Build history of the part. All positions in model axes, mm. A direction names the side the tool comes from. Round coordinates to 2 decimals unless told otherwise and drop trailing zeros. Order: outer loops, then holes, each group sorted by start corner. A loop starts at its lowest first (then second) coordinate and runs counter-clockwise, first axis right, second up. Notation, with made-up numbers: (79.25, -5.75) -> (98.25, -5.75) arc R24 cw to (98.25, 30.25) -> close; hole circle Ø9 at (-21, 74.25). An arc over 180 degrees is marked (long way). Answer as a JSON object with one key per item and string values.
from build123d import *

# Parameters (mm, degrees)
BOSS_EXTRUDE1_DEPTH = 4.5
SKETCH2_R           = 7.5
CUT_EXTRUDE1_DEPTH  = 50.942466899
SKETCH3_R           = 4
BOSS_EXTRUDE2_DEPTH = 7
BOSS_EXTRUDE3_DEPTH = 4.5
FILLET1_R           = 10
CUT_EXTRUDE4_DEPTH  = 62.754464971
SKETCH9_R           = 1
CUT_EXTRUDE5_DEPTH  = 62.182594482
SKETCH10_R          = 1.7
CUT_EXTRUDE6_DEPTH  = 2.4
CUT_EXTRUDE7_DEPTH  = 4.5
FILLET2_R           = 10
CUT_EXTRUDE8_DEPTH  = 51.658168147
SKETCH20_R          = 1
BOSS_EXTRUDE4_DEPTH = 4.5
SKETCH21_R          = 2
CUT_EXTRUDE9_DEPTH  = 3


with BuildPart() as part:
    # Sketch1 → Boss-Extrude1 (new body)
    with BuildSketch(Plane.XY):
        with BuildLine():
            Line((10.483870968, 22.695560128), (36.032258065, 10.893868862))
            ThreePointArc((36.032258065, 10.893868862), (43, 0), (36.032258065, -10.893868862))
            Line((36.032258065, -10.893868862), (10.483870968, -22.695560128))
            ThreePointArc((10.483870968, -22.695560128), (-25, 0), (10.483870968, 22.695560128))
        make_face()
    extrude(amount=BOSS_EXTRUDE1_DEPTH)

    # Sketch2 → Cut-Extrude1 (cut, through all)
    with BuildSketch(Plane.XY.offset(4.5)):
        with Locations((31, 0)):
            Circle(SKETCH2_R)
    extrude(amount=-CUT_EXTRUDE1_DEPTH, mode=Mode.SUBTRACT)

    # Sketch3 → Boss-Extrude2 (add)
    with BuildSketch(Plane.XY.offset(4.5)):
        Circle(SKETCH3_R)
    extrude(amount=BOSS_EXTRUDE2_DEPTH)

    # Sketch4 → Boss-Extrude3 (add)
    with BuildSketch(Plane(origin=(0, 0, 0), x_dir=(-1, 0, 0), z_dir=(0, 0, -1))):
        with BuildLine():
            Line((-36.032258065, 10.893868862), (-56.032258065, 10.893868862))
            Line((-56.032258065, 10.893868862), (-56.032258065, -10.893868862))
            Line((-56.032258065, -10.893868862), (-36.032258065, -10.893868862))
            ThreePointArc((-36.032258065, -10.893868862), (-43, 0), (-36.032258065, 10.893868862))
        make_face()
        with BuildLine():
            Line((22.501635968, 10.893868862), (42.501635968, 10.893868862))
            Line((42.501635968, 10.893868862), (42.501635968, -10.893868862))
            Line((42.501635968, -10.893868862), (22.501635968, -10.893868862))
            ThreePointArc((22.501635968, -10.893868862), (25, 0), (22.501635968, 10.893868862))
        make_face()
    extrude(amount=-BOSS_EXTRUDE3_DEPTH)

    # Fillet1
    fillet1_edges = [part.edges().sort_by_distance(p)[0] for p in [
        (56.032258065, 10.893868862, 2.25),
        (56.032258065, -10.893868862, 2.25),
        (-42.501635968, -10.893868862, 2.25),
        (-42.501635968, 10.893868862, 2.25),
    ]]
    fillet(fillet1_edges, radius=FILLET1_R)

    # Sketch8 → Cut-Extrude4 (cut, through all)
    with BuildSketch(Plane.XY.offset(4.5)):
        with BuildLine():
            Line((56.032258065, 0.893868862), (56.032258065, -0.893868862))
            ThreePointArc((56.032258065, -0.893868862), (55.873267798, -2.669967796), (55.401352579, -4.389590243))
            Line((55.401352579, -4.389590243), (55.401352579, 4.389590243))
            ThreePointArc((55.401352579, 4.389590243), (55.873267798, 2.669967796), (56.032258065, 0.893868862))
        make_face()
        with BuildLine():
            Line((-42.501635968, -0.893868862), (-42.501635968, 0.893868862))
            ThreePointArc((-42.501635968, 0.893868862), (-42.342645701, 2.669967796), (-41.870730482, 4.389590243))
            Line((-41.870730482, 4.389590243), (-41.870730482, -4.389590243))
            ThreePointArc((-41.870730482, -4.389590243), (-42.342645701, -2.669967796), (-42.501635968, -0.893868862))
        make_face()
    extrude(amount=-CUT_EXTRUDE4_DEPTH, mode=Mode.SUBTRACT)

    # Sketch9 → Cut-Extrude5 (cut, through all)
    with BuildSketch(Plane.XY.offset(4.5)):
        with Locations((-8.154330676, 12.589951995)):
            Circle(SKETCH9_R)
        with Locations((12.589951995, 8.154330676)):
            Circle(SKETCH9_R)
        with Locations((8.154330676, -12.589951995)):
            Circle(SKETCH9_R)
        with Locations((-12.589951995, -8.154330676)):
            Circle(SKETCH9_R)
    extrude(amount=-CUT_EXTRUDE5_DEPTH, mode=Mode.SUBTRACT)

    # Sketch10 → Cut-Extrude6 (cut)
    with BuildSketch(Plane.XY.offset(4.5)):
        with Locations((-8.154330676, 12.589951995)):
            Circle(SKETCH10_R)
        with Locations((12.589951995, 8.154330676)):
            Circle(SKETCH10_R)
        with Locations((8.154330676, -12.589951995)):
            Circle(SKETCH10_R)
        with Locations((-12.589951995, -8.154330676)):
            Circle(SKETCH10_R)
    extrude(amount=-CUT_EXTRUDE6_DEPTH, mode=Mode.SUBTRACT)

    # Sketch11 → Cut-Extrude7 (cut)
    with BuildSketch(Plane(origin=(0, 0, 0), x_dir=(-1, 0, 0), z_dir=(0, 0, -1))):
        with BuildLine():
            Line((-40.960235838, 14.646128502), (-73.67178465, 18.9155259))
            Line((-73.67178465, 18.9155259), (-68.640309048, -15.675868866))
            Line((-68.640309048, -15.675868866), (-41.444996676, -13.212200821))
            ThreePointArc((-41.444996676, -13.212200821), (-43.493415761, 0.756825882), (-40.960235838, 14.646128502))
        make_face()
    extrude(amount=-CUT_EXTRUDE7_DEPTH, mode=Mode.SUBTRACT)

    # Fillet2
    # the kernel refuses this fillet: 10 mm, written as the material it takes off along each edge
    with BuildSketch(Plane(origin=(42.113817462, -10.893868862, 28.001897109), x_dir=(0.1443560651040101, 0.9895258088941827, 0), z_dir=(0, 0, -1))) as fillet2_piece_1:
        with BuildLine():
            CenterArc((8.32021185, -9.941449502), FILLET2_R, 83.796810377, 73.10182949)
            Line((-0.877909984, -6.017859982), (-1.061872421, -5.939388192))
            ThreePointArc((-1.061872421, -5.939388192), (-0.636860154, -2.980058778), (-0.197905162, 0.028871213))
            Line((-0.197905162, 0.028871213), (-0.02161094, 0.19882899))
            ThreePointArc((-0.02161094, 0.19882899), (4.700379422, 0.454694668), (9.422369784, 0.19882899))
            Line((9.422369784, 0.19882899), (9.400758844, 0))
        make_face()
    extrude(amount=51.503794219, mode=Mode.SUBTRACT)
    with BuildSketch(Plane(origin=(42.113817462, 10.893868862, 28.001897109), x_dir=(-1, 0, 0), z_dir=(0, 0, -1))) as fillet2_piece_2:
        with BuildLine():
            CenterArc((8.636247816, -9.668172893), FILLET2_R, 104.801368002, 73.10182949)
            Line((-1.357056556, -9.302293499), (-1.556922643, -9.294975911))
            ThreePointArc((-1.556922643, -9.294975911), (-1.128460387, -4.585508816), (-0.193626747, 0.050086753))
            Line((-0.193626747, 0.050086753), (0, 0.2))
            ThreePointArc((0, 0.2), (3.040779699, 0.2), (6.030465629, 0.193363458))
            Line((6.030465629, 0.193363458), (6.081559398, 0))
        make_face()
    extrude(amount=51.503794219, mode=Mode.SUBTRACT)

    # Sketch12 → Cut-Extrude8 (cut, through all)
    with BuildSketch(Plane.XY.offset(4.5)):
        with BuildLine():
            Line((-22.501635968, 10.893868862), (-42.592674389, 14.819498464))
            Line((-42.592674389, 14.819498464), (-48.148078041, -13.612584929))
            Line((-48.148078041, -13.612584929), (-27.427309778, -14.315310761))
            Line((-27.427309778, -14.315310761), (-22.501635968, -10.893868862))
            ThreePointArc((-22.501635968, -10.893868862), (-25, 0), (-22.501635968, 10.893868862))
        make_face()
    extrude(amount=-CUT_EXTRUDE8_DEPTH, mode=Mode.SUBTRACT)

    # Sketch20 → Boss-Extrude4 (add)
    with BuildSketch(Plane.XY.offset(4.5)):
        with BuildLine():
            Line((55.798644786, -13.311457412), (55.798644786, 13.726073795))
            Line((55.798644786, 13.726073795), (30.798644786, 13.726073795))
            Line((30.798644786, 13.726073795), (30.798644786, 13.311457412))
            Line((30.798644786, 13.311457412), (36.032258065, 10.893868862))
            ThreePointArc((36.032258065, 10.893868862), (41.287575846, 7.470998455), (43.470874018, 1.591575362))
            ThreePointArc((43.470874018, 1.591575362), (43.5, 0), (43.470874018, -1.591575362))
            ThreePointArc((43.470874018, -1.591575362), (41.287575846, -7.470998455), (36.032258065, -10.893868862))
            Line((36.032258065, -10.893868862), (30.798644786, -13.311457412))
            Line((30.798644786, -13.311457412), (55.798644786, -13.311457412))
        make_face()
        with Locations((47.197816856, -7.773648876)):
            Circle(SKETCH20_R, mode=Mode.SUBTRACT)
        with Locations((47.197816856, 8.226351124)):
            Circle(SKETCH20_R, mode=Mode.SUBTRACT)
    extrude(amount=-BOSS_EXTRUDE4_DEPTH)

    # Sketch21 → Cut-Extrude9 (cut)
    with BuildSketch(Plane.XY.offset(4.5)):
        with Locations((47.197816856, 8.226351124)):
            Circle(SKETCH21_R)
        with Locations((47.197816856, -7.773648876)):
            Circle(SKETCH21_R)
    extrude(amount=-CUT_EXTRUDE9_DEPTH, mode=Mode.SUBTRACT)


solid = part.part
1) Cut at B-B, the plane x = 27.5. Give the cut face in (y, z).
Checked values:
{"outline": "(-14.84, 0) -> (-6.63, 0) -> (-6.63, 4.5) -> (-14.84, 4.5) -> close; (6.63, 0) -> (14.84, 0) -> (14.84, 4.5) -> (6.63, 4.5) -> close"}
2) Probe L1, parallel to X at y = 13.5, z = 1; L2, parallel to X at y = 9, z = 1.25; L3, parallel to Y at x = 31, z = 1.1. List the from-to ranges inside material, lowest first. Write a range as from..to.
Checked values:
{"L1": "x = -21.04..-8.57, -7.74..30.39, 30.8..55.8", "L2": "x = -23.32..12.06, 13.12..46.56, 47.83..55.8", "L3": "y = -13.31..-7.5, 7.5..13.73"}
3) Pull direction X, two halves, no side cores. Call faces 1 (the face through (-0.867, -3.905, 7.951)), 2 (the face through (10.89, 8.23, 3.32)), 3 (the face through (15, 0, 4.5)): pulls with the +X half, pulls with the -X half, needs draft (parallel to the pull), parting line crosses it, or undercut.
Checked values:
{"face 1": "parting line crosses it", "face 2": "undercut", "face 3": "needs draft"}
4) Cut at A-A, the plane y = 0. Give the cut face in (x, z), plus the area to 3 significant figures.
Checked values:
{"outline": "(-25, 0) -> (23.5, 0) -> (23.5, 4.5) -> (4, 4.5) -> (4, 11.5) -> (-4, 11.5) -> (-4, 4.5) -> (-25, 4.5) -> close; (38.5, 0) -> (55.8, 0) -> (55.8, 4.5) -> (38.5, 4.5) -> close", "area": "352 mm²"}
5) Cut at C-C, the plane z = 3. Give the cut face in (x, y), plus the area to 3 significant figures.
Checked values:
{"outline": "(10.48, -22.7) -> (30.8, -13.31) -> (55.8, -13.31) -> (55.8, 13.73) -> (30.8, 13.73) -> (30.8, 13.31) -> (10.48, 22.7) arc R25 ccw (long way) to start; hole circle Ø3.4 at (-12.59, -8.15); hole circle Ø3.4 at (-8.15, 12.59); hole circle Ø3.4 at (8.15, -12.59); hole circle Ø3.4 at (12.59, 8.15); hole circle Ø15 at (31, 0); hole circle Ø4 at (47.2, -7.77); hole circle Ø4 at (47.2, 8.23)", "area": "2,660 mm²"}
6) Cut at D-D, the plane x = 0. Give the cut face in (y, z).
Checked values:
{"outline": "(-25, 0) -> (25, 0) -> (25, 4.5) -> (4, 4.5) -> (4, 11.5) -> (-4, 11.5) -> (-4, 4.5) -> (-25, 4.5) -> close"}
7) Which spindle directions (+Z, -Z, +X, -X, +Y, -Y) get a long thin tool onto all of the face, cutting with end or side? Do faces 4 (the face through (-8.285, 13.581, 1.065)), 5 (the face through (43, -13.311, 2)), 6 (the face through (46.764, -9.726, 3.021)), 7 (the face through (43, 13.726, 2)). Say none if no direction does.
Checked values:
{"face 4": "+Z, -Z", "face 5": "+Z, -Z, +X, -Y", "face 6": "+Z", "face 7": "+Z, -Z, +X, +Y"}
8) Flat gauge pins, fed straight in: pin 1 Ø2.5 at (x, y) = (47.2, -7.77) entering from +Z; pin 2 Ø6 at (x, y) = (5, 18.5) entering from +Z; pin 3 Ø1.6 at (x, y) = (12.59, 8.15) entering from -Z; pin 4 Ø12 at (x, y) = (24.5, -19) entering from -Z. Where does each tip first touch, or does it go through?
Checked values:
{"pin 1": "stops at z = 1.5", "pin 2": "stops at z = 4.5", "pin 3": "passes through", "pin 4": "stops at z = 0"}
